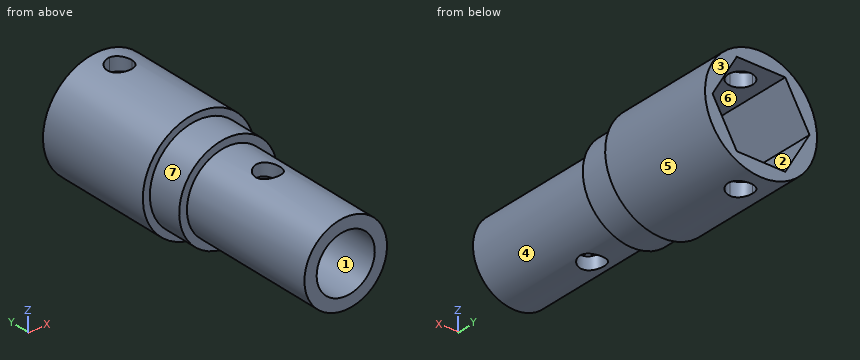
```python
from build123d import *

# Parameters (mm, degrees)
SKETCH1_R               = 8
BOSS_EXTRUDE1_DEPTH     = 17
CUT_EXTRUDE2_DEPTH      = 24.430749028
CUT_EXTRUDE2_DEPTH_BACK = 24.430749028
SKETCH3_R               = 5.900211262
SKETCH3_R_2             = 4.15
BOSS_EXTRUDE2_DEPTH     = 25
CUT_EXTRUDE3_DEPTH      = 28.440845526
CUT_EXTRUDE3_DEPTH_BACK = 28.440845526
SKETCH4_R               = 1.75
SKETCH5_R               = 7
SKETCH5_R_2             = 5.900211262
BOSS_EXTRUDE3_DEPTH     = 5


with BuildPart() as part:
    # Sketch1 → Boss-Extrude1 (new body)
    with BuildSketch(Plane.XZ):
        with Locations(Location((0, 0, 0), (0, 0, 270))):
            Circle(SKETCH1_R)
        Polygon((6.92820323, 0), (3.464101615, 6), (-3.464101615, 6), (-6.92820323, 0), (-3.464101615, -6), (3.464101615, -6), align=None, mode=Mode.SUBTRACT)
    extrude(amount=-BOSS_EXTRUDE1_DEPTH)

    # Sketch2 → Cut-Extrude2 (cut, two sides: drawn at the far end of the back side and taken through both)
    with BuildSketch(Plane.XY.offset(-6).offset(-CUT_EXTRUDE2_DEPTH_BACK)):
        with BuildLine():
            ThreePointArc((-1.75, 13.5), (-1.237436867, 12.262563133), (0, 11.75))
            ThreePointArc((0, 11.75), (1.237436867, 12.262563133), (1.75, 13.5))
            ThreePointArc((1.75, 13.5), (1.237436867, 14.737436867), (0, 15.25))
            ThreePointArc((0, 15.25), (-1.237436867, 14.737436867), (-1.75, 13.5))
        make_face()
    extrude(amount=CUT_EXTRUDE2_DEPTH + CUT_EXTRUDE2_DEPTH_BACK, mode=Mode.SUBTRACT)



with BuildPart() as body_2:
    # Sketch3 → Boss-Extrude2 (new body)
    with BuildSketch(Plane.XZ):
        with Locations(Location((0, 0, 0), (0, 0, 270))):
            Circle(SKETCH3_R)
        with Locations(Location((0, 0, 0), (0, 0, 270))):
            Circle(SKETCH3_R_2, mode=Mode.SUBTRACT)
    extrude(amount=BOSS_EXTRUDE2_DEPTH)

    # Sketch4 → Cut-Extrude3 (cut, two sides: drawn at the far end of the back side and taken through both)
    with BuildSketch(Plane.XY.offset(-CUT_EXTRUDE3_DEPTH_BACK)):
        with Locations((0, -11.75)):
            Circle(SKETCH4_R)
    extrude(amount=CUT_EXTRUDE3_DEPTH + CUT_EXTRUDE3_DEPTH_BACK, mode=Mode.SUBTRACT)


with BuildPart() as part_1:
    add(part.part)

    add(body_2.part)  # Boss-Extrude3 merges body 2
    # Sketch5 → Boss-Extrude3 (add)
    with BuildSketch(Plane.XZ):
        with Locations(Location((0, 0, 0), (0, 0, 270))):
            Circle(SKETCH5_R)
        with Locations(Location((0, 0, 0), (0, 0, 270))):
            Circle(SKETCH5_R_2, mode=Mode.SUBTRACT)
    extrude(amount=BOSS_EXTRUDE3_DEPTH)


solid = part_1.part
```
Input: part model. Units: mm. Frame: model coordinates. Face numbers are marked on the shaded views. A direction names the side the tool comes from. Coordinates: 2 decimals unless noted, no trailing zeros. Write each loop counter-clockwise with the first axis right and the second up, starting at its lowest first coordinate (ties: lowest second). Pieces come first, ordered by that corner, then holes.
1) Section C-C on z = 6.5. Output: boundary loops of the cut face in (x, y), and give its area (3 significant figures).
2) Mould query, pull axis X, two halves, no side actions, for the marked faces 1, 2, 3 and 4. Classes: pulls with the +X half, pulls with the -X half, needs draft (parallel to the pull), parting line crosses it, or undercut.
3) Section D-D on z = -2.25. Output: boundary loops of the cut face in (x, y), and give its area (3 significant figures).
4) Pin query (flat end, axial travel): pin 1 Ø2 at (x, z) = (1, -4) entering from +Y; pin 2 Ø2 at (x, y) = (-1, 6.5) entering from +Z; pin 3 Ø3 at (y, z) = (-10, 4.5) entering from +X; pin 4 Ø2 at (x, y) = (0, -11.75) entering from -Z. Return the tip coordinate at first contact, or that it passes through.
5) Section A-A on y = 0.5. Output: boundary loops of the cut face in (x, z), and give its area (3 significant figures).
6) Section B-B on y = -11.75. Output: boundary loops of the cut face in (x, z).
7) Material intervals for line 1 along X through (y, z) = (-19, 0); line 2 along Y through (x, z) = (0, -4.6), sorted ascending.
8) Set-up query: the marked faces 5, 6 and 7. Return all of +Z, -Z, +X, -X, +Y, -Y with unobstructed straight access to the full face (end or side cutting, diameter ignored); none if empty.
Check result:
1. outline: (-4.66, 0) - (-2.6, 0) - (-2.6, -5) - (2.6, -5) - (2.6, 0) - (4.66, 0) - (4.66, 17) - (-4.66, 17) - close; hole circle Ø3.5 at (0, 13.5)
1. area: 175 mm2
2. face 1: undercut
2. face 2: undercut
2. face 3: needs draft
2. face 4: parting line crosses it
3. outline: (-7.68, 0) - (-6.63, 0) - (-6.63, -5) - (-5.45, -5) - (-5.45, -25) - (-3.49, -25) - (-3.49, 0) - (-5.63, 0) - (-5.63, 17) - (-7.68, 17) - close; (3.49, -25) - (5.45, -25) - (5.45, -5) - (6.63, -5) - (6.63, 0) - (7.68, 0) - (7.68, 17) - (5.63, 17) - (5.63, 0) - (3.49, 0) - close
3. area: 180 mm2
4. pin 1: stops at y = 0
4. pin 2: stops at z = 8
4. pin 3: stops at x = 5.08
4. pin 4: passes through
5. outline: circle Ø16 at (0, 0); hole (-6.93, 0) - (-3.46, -6) - (3.46, -6) - (6.93, 0) - (3.46, 6) - (-3.46, 6) - close
5. area: 76.4 mm2
6. outline: (-1.75, -5.63) - (-1.75, -3.76) arc R4.15 cw to (-1.75, 3.76) - (-1.75, 5.63) arc R5.9 ccw to start; (1.75, -5.63) arc R5.9 ccw to (1.75, 5.63) - (1.75, 3.76) arc R4.15 cw to (1.75, -3.76) - close
7. line 1: x = -5.9 to -4.15, 4.15 to 5.9
7. line 2: y = -25 to -13.5, -10 to 0
8. face 5: +Y, -Y
8. face 6: +Y
8. face 7: -Y
